```python
from build123d import *

# Parameters (mm, degrees)
F1_DEPTH = 65
F3_W     = 40.1219656318
F3_H     = 20.9779888391
F3_W_2   = 49.7560687363
F3_H_2   = 38.9171534163
F3_H_3   = 18.6112551019
F4_DEPTH = 77.8353068326
F5_R     = 15
F6_DEPTH = 130.001


with BuildPart() as f1:
    # F0 (on Front) → F1 (new body, symmetric)
    with BuildSketch(Plane.XZ):
        with BuildLine():
            Line((38.9171534163, -50.8422553539), (38.9171534163, 0))
            ThreePointArc((38.9171534163, 0), (0, 38.9171534163), (-38.9171534163, 0))
            Line((-38.9171534163, 0), (-38.9171534163, -50.8422553539))
            Line((-38.9171534163, -50.8422553539), (38.9171534163, -50.8422553539))
        make_face()
    extrude(amount=F1_DEPTH, both=True)

    # F3 (on face) → F4 (cut, through all)
    with BuildSketch(Plane.YZ.offset(38.9171534163)):
        with Locations((-44.9390171841, -40.3532609344)):
            Rectangle(F3_W, F3_H)
        with Locations((44.9390171841, -40.3532609344)):
            Rectangle(F3_W, F3_H)
        with Locations((0, 19.4585767082)):
            Rectangle(F3_W_2, F3_H_2)
        with Locations((0, -9.3056275509)):
            Rectangle(F3_W_2, F3_H_3)
    extrude(amount=-F4_DEPTH, mode=Mode.SUBTRACT)

    # F5 (on face) → F6 (cut, through all)
    with BuildSketch(Plane.XZ.offset(65)):
        Circle(F5_R)
    extrude(amount=-F6_DEPTH, mode=Mode.SUBTRACT)


solid = f1.part
```
The model under review builds one solid part; all positions refer to its coordinate system, in mm. A direction names the side the tool comes from. Coordinates: 2 decimals unless noted, no trailing zeros. Order: outer loops, then holes, each group sorted by start corner. A loop starts at its lowest first (then second) coordinate and runs counter-clockwise, first axis right, second up. Notation, with made-up numbers: (75.25, 29) -> (132.25, 29) arc R28 cw to (132.25, 65) -> close; hole circle Ø4 at (-9, 37). An arc over 180 degrees is marked (long way). Answer in a Markdown table with one row per item. Add a question column.
Item 1: We need section B-B on x = 0. Write out the cut boundary in (y, z), plus the area to 3 significant figures.
Item 2: Machinability: for faces 1 (the flat face through (1, -24.878, 17)), 2 (the flat face through (1, 45, -29.864)), 3 (the flat face through (1, -45, -29.864)), which of the approach directions +Z, -Z, +X, -X, +Y, -Y give a long, thin tool a straight path to every point of the face, cutting with its end or side? Answer none if there is none.
Item 3: Clearance check with flat-ended pins moving along their axes: pin 1 (20 mm diameter, centred on x = -18.5, y = 47.5, fed in from -Z); pin 2 (17.5 mm diameter, centred on x = -7.5, z = 4, fed in from -Y); pin 3 (12 mm diameter, centred on x = 10.5, y = 48.5, fed in from +Z); pin 4 (1.5 mm diameter, centred on x = 12, z = -35, fed in from -Y). State where each tip first meets the part, or that it passes through.
Item 4: To check wall thickness, follow probe 1 along Y at (x, z) = (22.5, -3.5); probe 2 along Z at (x, y) = (0, 42); probe 3 along X at (y, z) = (-58, 12). State the ranges of each line that lie inside material, in increasing order.
Item 5: Mouldability with a two-part tool opening along X and no side actions: class faces 4 (the flat face through (1, 24.878, -41)), 5 (the cylindrical face through (0.856, -45.22, 38.908)), 6 (the cylindrical face through (-14.985, -45.22, 0.66)) as +X half, -X half, draft (parallel to the pull), parting line (faces both ways), or undercut.
Item 6: We need section C-C on z = 33. Write out the cut boundary in (x, y).
Item 7: We need section A-A on z = 13.5. Write out the cut boundary in (x, y).
Item 8: We need section D-D on y = 51. Write out the cut boundary in (x, z), plus the area to 3 significant figures.
Final values:
| question | item | result |
|---|---|---|
| 1 | outline | (-65, -29.86) -> (-24.88, -29.86) -> (-24.88, -50.84) -> (24.88, -50.84) -> (24.88, -29.86) -> (65, -29.86) -> (65, -15) -> (24.88, -15) -> (24.88, -18.61) -> (-24.88, -18.61) -> (-24.88, -15) -> (-65, -15) -> close; (-65, 15) -> (-24.88, 15) -> (-24.88, 38.92) -> (-65, 38.92) -> close; (24.88, 15) -> (65, 15) -> (65, 38.92) -> (24.88, 38.92) -> close |
| 1 | area | 4,720 mm2 |
| 2 | face 1 | +Z, +X, -X |
| 2 | face 2 | -Z, +X, -X, +Y |
| 2 | face 3 | -Z, +X, -X, -Y |
| 3 | pin 1 | stops at z = -29.86 |
| 3 | pin 2 | stops at y = -65 |
| 3 | pin 3 | stops at z = 38.66 |
| 3 | pin 4 | stops at y = -24.88 |
| 4 | probe 1 | y = -65 to -24.88, 24.88 to 65 |
| 4 | probe 2 | z = -29.86 to -15, 15 to 38.92 |
| 4 | probe 3 | x = -37.02 to -9, 9 to 37.02 |
| 5 | face 4 | draft |
| 5 | face 5 | parting line |
| 5 | face 6 | undercut |
| 6 | outline | (-20.63, -65) -> (20.63, -65) -> (20.63, -24.88) -> (-20.63, -24.88) -> close; (-20.63, 24.88) -> (20.63, 24.88) -> (20.63, 65) -> (-20.63, 65) -> close |
| 7 | outline | (-36.5, -65) -> (-6.54, -65) -> (-6.54, -24.88) -> (-36.5, -24.88) -> close; (-36.5, 24.88) -> (-6.54, 24.88) -> (-6.54, 65) -> (-36.5, 65) -> close; (6.54, -65) -> (36.5, -65) -> (36.5, -24.88) -> (6.54, -24.88) -> close; (6.54, 24.88) -> (36.5, 24.88) -> (36.5, 65) -> (6.54, 65) -> close |
| 8 | outline | (-38.92, -29.86) -> (38.92, -29.86) -> (38.92, 0) arc R38.92 ccw to (-38.92, 0) -> close; hole circle Ø30 at (0, 0) |
| 8 | area | 4,000 mm2 |
